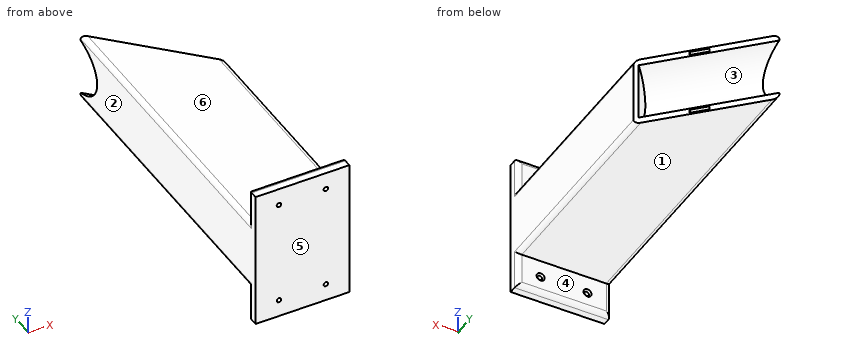
from build123d import *

# Parameters (mm, degrees)
SKETCH1_W                                         = 50.8
SKETCH1_H                                         = 76.2
BOSS_EXTRUDE1_DEPTH                               = 6.35
SKETCH2_W                                         = 50.8
SKETCH2_H                                         = 38.1
BOSS_EXTRUDE2_DEPTH                               = 171.6066
CUT_EXTRUDE1_DEPTH                                = 183.535025619
CUT_EXTRUDE1_DEPTH_BACK                           = 183.535025619
BOSS_EXTRUDE3_REACH                               = 237.296
SKETCH20_W                                        = 38.1
SKETCH20_H                                        = 2.54
BOSS_EXTRUDE4_REACH                               = 129.523
CSK_FOR_2_FLAT_HEAD_MACHINE_SCREW_100_D           = 2.4384
CSK_FOR_2_FLAT_HEAD_MACHINE_SCREW_100_CSINK_D     = 4.3688
CSK_FOR_2_FLAT_HEAD_MACHINE_SCREW_100_CSINK_ANGLE = 100
FILLET1_R                                         = 2.54
FILLET2_R                                         = 2.54
SKETCH29_W                                        = 1.860730234
SKETCH29_H                                        = 10
CUT_EXTRUDE2_DEPTH                                = 30
CUT_EXTRUDE3_REACH                                = 232.917
CUT_EXTRUDE3_END_RADIUS                           = 19.51
SKETCH30_W                                        = 43.463948775
SKETCH30_H                                        = 25.418064868


with BuildPart() as part:
    # Sketch1 → Boss-Extrude1 (new body)
    with BuildSketch(Plane(origin=(0, 0, 0), x_dir=(1, 0, 0), z_dir=(0, 1, 0))):
        with Locations((-132.195454545, 0)):
            Rectangle(SKETCH1_W, SKETCH1_H)
    extrude(amount=BOSS_EXTRUDE1_DEPTH)

    # Sketch2 → Boss-Extrude2 (add)
    with BuildSketch(Plane(origin=(0, 6.35, 0), x_dir=(1, 0, 0), z_dir=(0, 1, 0))):
        with Locations((-132.195454545, 0)):
            Rectangle(SKETCH2_W, SKETCH2_H)
    extrude(amount=BOSS_EXTRUDE2_DEPTH)

    # Sketch19 → Cut-Extrude1 (cut, two sides: drawn at the far end of the back side and taken through both)
    with BuildSketch(Plane(origin=(-167.776027273, 167.776027273, 0), x_dir=(-0.7071067811865488, -0.7071067811865462, 0), z_dir=(0.7071067811865462, -0.7071067811865488, 0)).offset(-CUT_EXTRUDE1_DEPTH_BACK)):
        with BuildLine():
            Line((-14.397504024, 16.51), (-14.397504024, -16.51))
            ThreePointArc((-14.397504024, -16.51), (2.112495976, 0), (-14.397504024, 16.51))
        make_face()
    extrude(amount=CUT_EXTRUDE1_DEPTH + CUT_EXTRUDE1_DEPTH_BACK, mode=Mode.SUBTRACT)

    # SurfaceCut1
    split(bisect_by=Plane(origin=(6.588470279, 6.588470279, 0), x_dir=(0, 0, 1), z_dir=(-0.7071067811865488, -0.7071067811865464, 0)), keep=Keep.TOP)

    # Sketch20 → Boss-Extrude3 (add, up to next)
    with BuildSketch(Plane(origin=(6.588470279, 6.588470279, 0), x_dir=(0, 0, -1), z_dir=(0.7071067811865487, 0.7071067811865465, 0)), mode=Mode.PRIVATE) as boss_extrude3_sk1:
        with Locations((0, 161.619084242)):
            Rectangle(SKETCH20_W, SKETCH20_H)
    boss_extrude3_tool1 = extrude(boss_extrude3_sk1.sketch, amount=-BOSS_EXTRUDE3_REACH, mode=Mode.PRIVATE) - part.part
    add(boss_extrude3_tool1.solids().sort_by_distance((-107.69348, 120.870421, 0))[0])

    # Boss-Extrude4: up to this face of the body (flat: up to its plane)
    boss_extrude4_end = Plane(part.part.faces().sort_by_distance((-106.795454545, 52.426789341, 0))[0])
    # Sketch22 → Boss-Extrude4 (add, up to the picked face)
    with BuildSketch(Plane(origin=(-113.383924824, 113.383924824, 0), x_dir=(0, 0, -1), z_dir=(0.7071067811865465, -0.7071067811865486, 0)), mode=Mode.PRIVATE) as boss_extrude4_sk1:
        with BuildLine():
            Line((-15.709032434, 9.317504024), (15.709032434, 9.317504024))
            ThreePointArc((15.709032434, 9.317504024), (0, -6.39152841), (-15.709032434, 9.317504024))
        make_face()
    boss_extrude4_tool1 = split(extrude(boss_extrude4_sk1.sketch, amount=BOSS_EXTRUDE4_REACH, mode=Mode.PRIVATE), bisect_by=boss_extrude4_end, keep=Keep.BOTH, mode=Mode.PRIVATE)
    add(boss_extrude4_tool1.solids().sort_by(Axis((-111.509821, 115.258029, 0), (0.7071067811865465, -0.7071067811865486, 0)))[0])

    # CSK for #2 Flat Head Machine Screw (100)1 (through all)
    with Locations(Plane(origin=(0, 6.35, 0), x_dir=(1, 0, 0), z_dir=(0, 1, 0))):
        with Locations((-144.895454545, -28.575), (-119.495454545, -28.575)):
            csk_for_2_flat_head_machine_screw_100 = CounterSinkHole(CSK_FOR_2_FLAT_HEAD_MACHINE_SCREW_100_D / 2, CSK_FOR_2_FLAT_HEAD_MACHINE_SCREW_100_CSINK_D / 2, counter_sink_angle=CSK_FOR_2_FLAT_HEAD_MACHINE_SCREW_100_CSINK_ANGLE)

    # Mirror1: CSK for #2 Flat Head Machine Screw (100)1 across plane
    add(csk_for_2_flat_head_machine_screw_100.mirror(Plane.XY), mode=Mode.SUBTRACT)

    # Fillet1
    fillet1_edges = [part.edges().sort_by_distance(p)[0] for p in [
        (-157.595454545, 88.561197552, 19.05),
        (-106.795454545, 63.161197552, 19.05),
        (-106.795454545, 63.161197552, -19.05),
        (-157.595454545, 88.561197552, -19.05),
    ]]
    fillet(fillet1_edges, radius=FILLET1_R)

    # Fillet2
    fillet2_edges = [part.edges().sort_by_distance(p)[0] for p in [
        (-157.595454545, 6.35, -27.305),
        (-132.195454545, 6.35, -38.1),
        (-106.795454545, 6.35, -27.305),
        (-157.595454545, 6.35, 27.305),
        (-132.195454545, 6.35, 38.1),
        (-106.795454545, 6.35, 27.305),
    ]]
    fillet(fillet2_edges, radius=FILLET2_R)

    # Sketch29 → Cut-Extrude2 (cut)
    with BuildSketch(Plane(origin=(6.588470279, 6.588470279, 0), x_dir=(0, 0, -1), z_dir=(0.7071067811865487, 0.7071067811865465, 0))):
        with Locations((17.36598973, 192.889084242)):
            Rectangle(SKETCH29_W, SKETCH29_H)
        with Locations((-17.36598973, 192.889084242)):
            Rectangle(SKETCH29_W, SKETCH29_H)
    extrude(amount=-CUT_EXTRUDE2_DEPTH, mode=Mode.SUBTRACT)

    # Cut-Extrude3: up to this cylinder (the profile starts outside it)
    cut_extrude3_end = Plane(origin=(-59.656167273, 80.017312727, 0), z_dir=(0.7071067811865462, -0.7071067811865488, 0)) * Cylinder(CUT_EXTRUDE3_END_RADIUS, 505.854, mode=Mode.PRIVATE)
    # Sketch30 → Cut-Extrude3 (cut, up to the surface)
    with BuildSketch(Plane(origin=(0, 6.35, 0), x_dir=(1, 0, 0), z_dir=(0, 1, 0)), mode=Mode.PRIVATE) as cut_extrude3_sk1:
        with Locations((-133.323480158, 0)):
            Rectangle(SKETCH30_W, SKETCH30_H)
    cut_extrude3_tool1 = extrude(cut_extrude3_sk1.sketch, amount=CUT_EXTRUDE3_REACH, mode=Mode.PRIVATE) - cut_extrude3_end
    add(cut_extrude3_tool1.solids().sort_by_distance((-133.32348, 6.35, 0))[0], mode=Mode.SUBTRACT)


solid = part.part
Model file for the job. Use its own axes, mm. Face numbers are marked on the shaded views. A direction names the side the tool comes from. Round coordinates to 2 decimals unless told otherwise and drop trailing zeros. Loops run counter-clockwise (first coordinate to the right, second up) from the corner with the lowest first, then second, coordinate; pieces in that order, holes last. Notation, with made-up numbers: (26.25, 86.5) -> (36.25, 86.5) arc R22 cw to (36.25, 99.5) -> close; hole circle Ø2 at (-30, 9.5). An arc over 180 degrees is marked (long way). Answer as CSV lines item,"result". Start each with the question number.
1) Slice it at B-B (z = -6). List the corners of the cut face in (x, y), plus the area to 3 significant figures.
2) Slice it at D-D (z = 5.5). List the corners of the cut face in (x, y), plus the area to 3 significant figures.
3) Slice it at C-C (x = -150.5). State how many separate pieces and enclosed holes the cut face has, plus the area to 3 significant figures.
4) Mould opens along Z. For the marked faces 1, 2 and 3 say: +Z half, -Z half, draft (parallel to the pull), parting line (faces both ways), or undercut.
5) Tool access for the marked faces 4, 5 and 6: list every direction of +Z, -Z, +X, -X, +Y, -Y with a clear straight run to the whole face (end or side of a thin tool).
6) Probe line 1 along Z through (x, y) = (-117, 88.5); line 2 along X through (y, z) = (20.5, -7); line 3 along Y through (x, z) = (-142.5, 10.5). List the from-to ranges inside material, lowest first.
7) Slice it at A-A (y = 25.5). List the corners of the cut face in (x, z).
8) Pin check, flat tips, straight feed: P1, Ø14, axis at x = -146.5, y = 131.5, coming from the +Z side; P2, Ø13, axis at x = -121, z = 27.5, coming from the +Y side; P3, Ø4, axis at y = 103, z = -19, coming from the +X side. Stop position of each tip, or through.
Filled in:
1,outline,"(-157.6, 0) -> (-106.8, 0) -> (-106.8, 119.97) -> (-108.59, 121.77) -> (-115.88, 114.48) -> (-157.6, 156.2) -> close; hole (-155.06, 6.35) -> (-111.59, 6.35) -> (-111.59, 105.7) -> (-155.06, 149.16) -> close"
1,area,"1,460 mm2"
2,outline,"(-157.6, 0) -> (-106.8, 0) -> (-106.8, 119.97) -> (-108.59, 121.77) -> (-116.01, 114.35) -> (-157.6, 155.94) -> close; hole (-155.06, 6.35) -> (-111.59, 6.35) -> (-111.59, 105.48) -> (-155.06, 148.94) -> close"
2,area,"1,460 mm2"
3,separate pieces,"1"
3,enclosed holes,"3"
3,area,"2,540 mm2"
4,face 1,"-Z half"
4,face 2,"draft"
4,face 3,"undercut"
5,face 4,"-Z, +X, -X, +Y"
5,face 5,"+Z, -Z, +X, -X, -Y"
5,face 6,"+Z, +X, -X, +Y"
6,line 1,"z = -19.05 to -12.71, 12.71 to 19.05"
6,line 2,"x = -157.6 to -155.06, -111.59 to -106.8"
6,line 3,"y = 0 to 6.35, 139.61 to 144.84"
7,outline,"(-157.6, -16.51) arc R2.54 ccw to (-155.06, -19.05) -> (-109.34, -19.05) arc R2.54 ccw to (-106.8, -16.51) -> (-106.8, 16.51) arc R2.54 ccw to (-109.34, 19.05) -> (-155.06, 19.05) arc R2.54 ccw to (-157.6, 16.51) -> close; hole (-155.06, -12.71) -> (-111.59, -12.71) -> (-111.59, 12.71) -> (-155.06, 12.71) -> close"
8,P1,"stops at z = 19.05"
8,P2,"stops at y = 6.35"
8,P3,"stops at x = -106.84"
